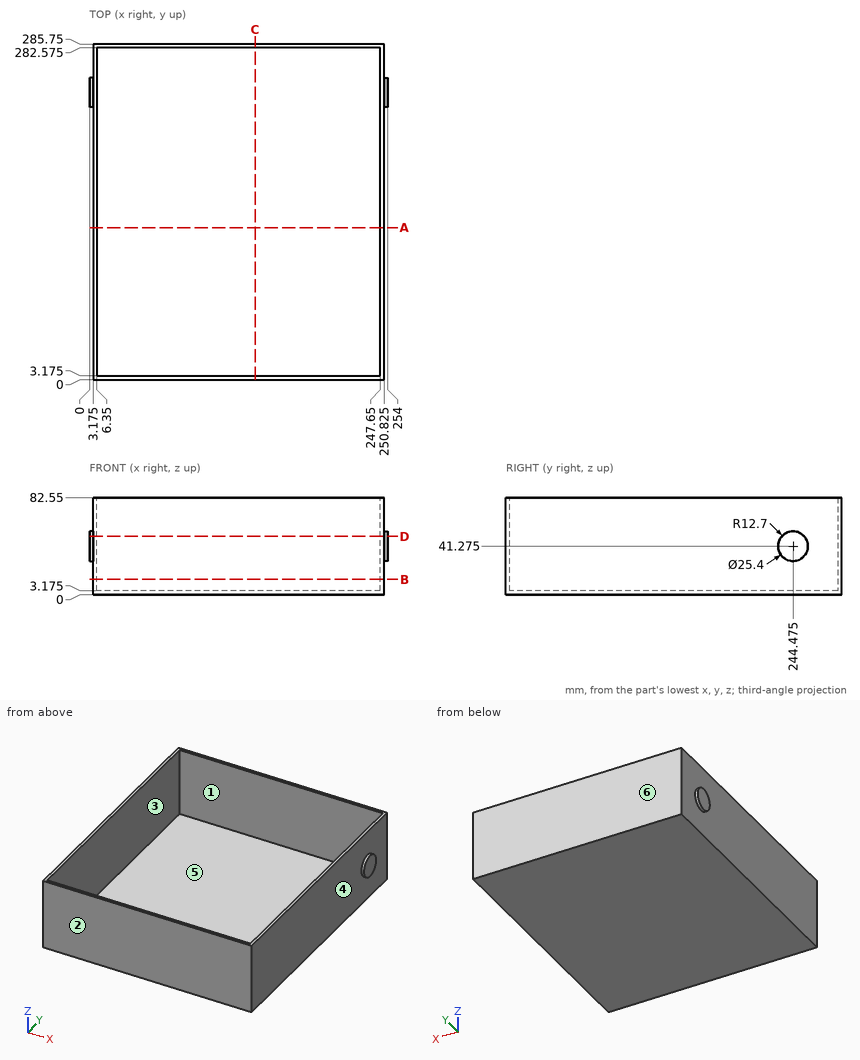
Drawing for the job (mm, zero at the part's lowest x, y, z). A direction names the side the tool comes from. Give positions to 0.01 mm unless a question says otherwise; leave off trailing zeros. Order: outer loops, then holes, each group sorted by start corner. A loop starts at its lowest first (then second) coordinate and runs counter-clockwise, first axis right, second up. Notation, with made-up numbers: (-11, -21.75) -> (44, -21.75) arc R18 ccw to (44, -4.75) -> close; hole circle Ø7 at (53, 14.25). An arc over 180 degrees is marked (long way). Use one line per item in the form item = value.
(1) Flat gauge pins, fed straight in: P1, Ø5, axis at y = 209.5, z = 43, coming from the -X side (3 decimals); P2, Ø8, axis at y = 40.5, z = 53, coming from the +X side (3 decimals); P3, Ø10, axis at x = 226.5, y = 187, coming from the +Z side (3 decimals). Where does each tip first touch, or does it go through?
Solution:
P1 = 3.175
P2 = 250.825
P3 = 3.175
(2) Saw through at D-D (z = 49.5). Write the cut outline in (x, y) (3 decimals).
Solution:
outline = (0, 234.798) -> (3.175, 234.798) -> (3.175, 0) -> (250.825, 0) -> (250.825, 234.798) -> (254, 234.798) -> (254, 254.152) -> (250.825, 254.152) -> (250.825, 285.75) -> (3.175, 285.75) -> (3.175, 254.152) -> (0, 254.152) -> close; hole (6.35, 3.175) -> (247.65, 3.175) -> (247.65, 282.575) -> (6.35, 282.575) -> close
(3) Tool access for the marked faces 5 and 6: list every direction of +Z, -Z, +X, -X, +Y, -Y with a clear straight run to the whole face (end or side of a thin tool).
Solution:
face_5 = +Z
face_6 = +Z, -Z, +X, -X, +Y
(4) Drill centre lines: line 1 (X direction, y = 223, z = 7.5) (3 decimals); line 2 (Y direction, x = 117, z = 27.5) (3 decimals); line 3 (Z direction, x = 228.5, y = 86) (3 decimals). Where is each one in solid material? Low to high. Write a range as from..to.
Solution:
line_1 = 3.175..6.35, 247.65..250.825
line_2 = 0..3.175, 282.575..285.75
line_3 = 0..3.175
(5) Saw through at C-C (x = 141). Write the cut outline in (y, z) (3 decimals).
Solution:
outline = (0, 0) -> (285.75, 0) -> (285.75, 82.55) -> (282.575, 82.55) -> (282.575, 3.175) -> (3.175, 3.175) -> (3.175, 82.55) -> (0, 82.55) -> close
(6) Saw through at A-A (y = 129.5). Write the cut outline in (x, z) (3 decimals), then the cut area to 3 significant figures.
Solution:
outline = (3.175, 0) -> (250.825, 0) -> (250.825, 82.55) -> (247.65, 82.55) -> (247.65, 3.175) -> (6.35, 3.175) -> (6.35, 82.55) -> (3.175, 82.55) -> close
area = 1,290 mm²
(7) Saw through at B-B (z = 13). Write the cut outline in (x, y) (3 decimals), then the cut area to 3 significant figures.
Solution:
outline = (3.175, 0) -> (250.825, 0) -> (250.825, 285.75) -> (3.175, 285.75) -> close; hole (6.35, 3.175) -> (247.65, 3.175) -> (247.65, 282.575) -> (6.35, 282.575) -> close
area = 3,350 mm²
(8) Pull direction Y, two halves, no side cores. Call the marked faces 1, 2, 3 and 4: +Y half, -Y half, draft (parallel to the pull), parting line (faces both ways), or undercut.
Solution:
face_1 = undercut
face_2 = -Y half
face_3 = undercut
face_4 = draft
